Part model, mm, in its own coordinate system. A direction names the side the tool comes from. Round coordinates to 2 decimals unless told otherwise and drop trailing zeros. Loops run counter-clockwise (first coordinate to the right, second up) from the corner with the lowest first, then second, coordinate; pieces in that order, holes last.
from build123d import *

# Parameters (mm, degrees)
BOSS_EXTRUDE1_DEPTH = 70
SKETCH2_W           = 20
SKETCH2_H           = 50
CUT_EXTRUDE1_DEPTH  = 50
SKETCH3_W           = 20
SKETCH3_H           = 26
CUT_EXTRUDE2_DEPTH  = 20


with BuildPart() as part:
    # Sketch1 → Boss-Extrude1 (new body)
    with BuildSketch(Plane.XY):
        Polygon((-33.026980357, 100.831089677), (-83.026980357, 100.831089677), (-83.026980357, 76.831089677), (-133.026980357, 76.831089677), (-133.026980357, 50.831089677), (-33.026980357, 50.831089677), align=None)
    extrude(amount=BOSS_EXTRUDE1_DEPTH)

    # Sketch2 → Cut-Extrude1 (cut)
    with BuildSketch(Plane.XY.offset(70)):
        with Locations((-43.026980357, 75.831089677)):
            Rectangle(SKETCH2_W, SKETCH2_H)
    extrude(amount=-CUT_EXTRUDE1_DEPTH, mode=Mode.SUBTRACT)

    # Sketch3 → Cut-Extrude2 (cut)
    with BuildSketch(Plane.XY.offset(70)):
        with Locations((-123.026980357, 63.831089677)):
            Rectangle(SKETCH3_W, SKETCH3_H)
    extrude(amount=-CUT_EXTRUDE2_DEPTH, mode=Mode.SUBTRACT)


solid = part.part
1) Drop flat-ended pins along their axis: pin 1 Ø15 at (y, z) = (70, 45) entering from +X; pin 2 Ø10 at (x, y) = (-126.5, 65.5) entering from +Z; pin 3 Ø12 at (y, z) = (86.5, 52) entering from -X. Give the stop position or say it passes through.
Values:
pin 1: stops at x = -53.03
pin 2: stops at z = 50
pin 3: stops at x = -83.03
2) Slice it at C-C, the plane x = -50.5. Give the cut face in (y, z), then the cut area to 3 significant figures.
Values:
outline: (50.83, 0) - (100.83, 0) - (100.83, 20) - (50.83, 20) - close
area: 1,000 mm2
3) Slice it at D-D, the plane y = 67.5. Give the cut face in (x, z), then the cut area to 3 significant figures.
Values:
outline: (-133.03, 0) - (-33.03, 0) - (-33.03, 20) - (-53.03, 20) - (-53.03, 70) - (-113.03, 70) - (-113.03, 50) - (-133.03, 50) - close
area: 5,600 mm2
4) Tool access for faces 1 (the face through (-123, 64, 50)), 2 (the face through (-33.027, 75, 10)), 3 (the face through (-43, 76, 20)): list every direction of +Z, -Z, +X, -X, +Y, -Y with a clear straight run to the whole face (end or side of a thin tool).
Values:
face 1: +Z, -X, +Y, -Y
face 2: +Z, -Z, +X, +Y, -Y
face 3: +Z, +X, +Y, -Y
5) Wall check: line 1 along Z through (x, y) = (-38, 60.5); line 2 along X through (y, z) = (65, 60); line 3 along X through (y, z) = (96.5, 58). Give the ranges that are in metal, low to high.
Values:
line 1: z = 0 to 20
line 2: x = -113.03 to -53.03
line 3: x = -83.03 to -53.03
6) Mould opens along Y. For faces 4 (the face through (-83.027, 89, 35)), 5 (the face through (-84, 50.831, 27)), 6 (the face through (-108, 76.831, 27)) say: released by +Y, released by -Y, zero draft, split by the parting line, or undercut.
Values:
face 4: zero draft
face 5: released by -Y
face 6: released by +Y
7) Slice it at A-A, the plane y = 89.5. Give the cut face in (x, z).
Values:
outline: (-83.03, 0) - (-33.03, 0) - (-33.03, 20) - (-53.03, 20) - (-53.03, 70) - (-83.03, 70) - close
8) Slice it at B-B, the plane z = 15. Give the cut face in (x, y).
Values:
outline: (-133.03, 50.83) - (-33.03, 50.83) - (-33.03, 100.83) - (-83.03, 100.83) - (-83.03, 76.83) - (-133.03, 76.83) - close
